Check sheet for the drawn part. Datum: minimum x, y, z corner. Units: mm. A direction names the side the tool comes from. Coordinates: 2 decimals unless noted, no trailing zeros. Order: outer loops, then holes, each group sorted by start corner. A loop starts at its lowest first (then second) coordinate and runs counter-clockwise, first axis right, second up. Notation, with made-up numbers: M 69.5,23 L 102.5,23 A30 cw 102.5,50 Z; hole C -23,-8.75 d8. An arc over 180 degrees is marked long. Answer in a Markdown table with one row per item. Add a question column.
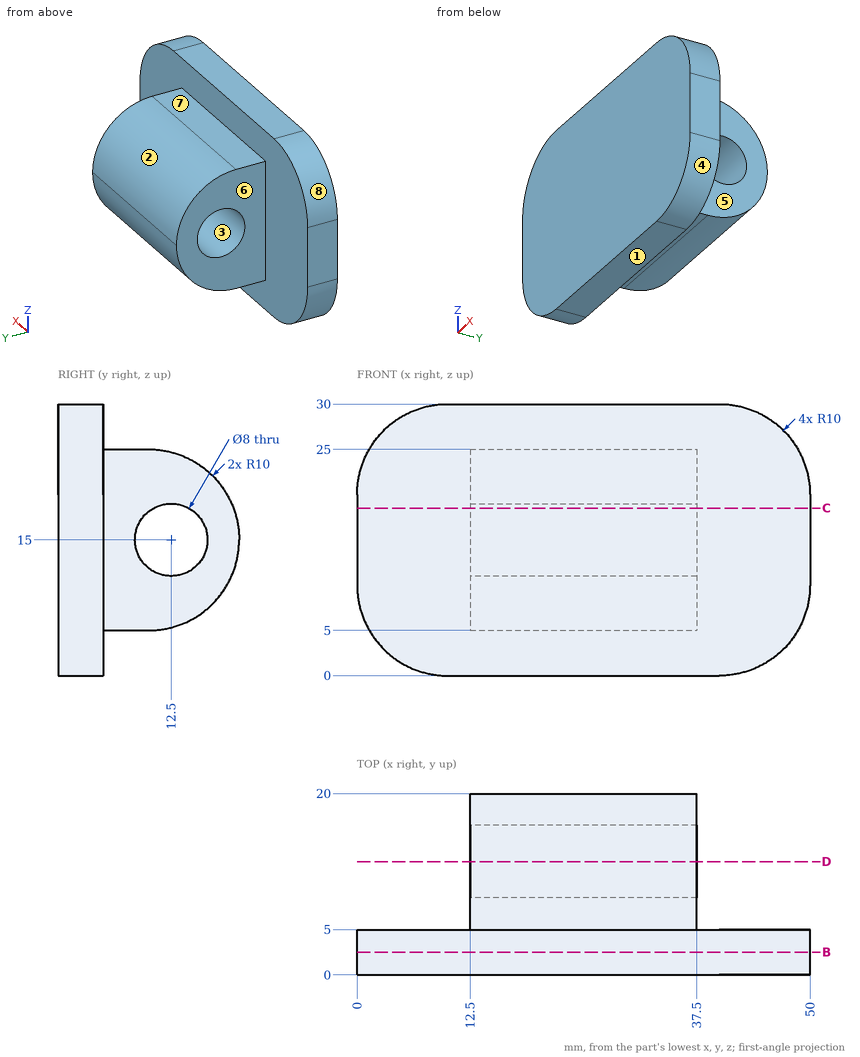
1. Scan lines: line 1 (Y direction, x = 18.25, z = 15); line 2 (X direction, y = 13, z = 9.5); line 3 (Y direction, x = 47, z = 17). Record each from-to range of solid material in increasing order.
2. Section check B-B on y = 2.5. Enter the section's corners in (x, z), then the cut area to 3 significant figures.
3. Section check D-D on y = 12.5. Enter the section's corners in (x, z), then the cut area to 3 significant figures.
4. Release check for a two-part mould opening along Y. For the marked faces 1, 2 and 3 record: released by +Y, released by -Y, zero draft, split by the parting line, or undercut.
5. Section check C-C on z = 18.5. Enter the section's corners in (x, y), then the cut area to 3 significant figures.
6. Go/stop test with flat-tipped pins: pin 1 Ø10 at (x, y) = (5.5, 10.5) entering from +Z; pin 2 Ø4 at (y, z) = (9, 20.5) entering from -X; pin 3 Ø1.5 at (x, y) = (31, 7.5) entering from +Z; pin 4 Ø7.5 at (y, z) = (9, 15.5) entering from +X. Record where each tip stops, or that it passes through.
7. Set-up check for the marked faces 4, 5, 6, 7 and 8: record each of +Z, -Z, +X, -X, +Y, -Y from which the full face is reachable in a straight line by a thin tool's end or side.
Result sheet:
| question | item | result |
|---|---|---|
| 1 | line 1 | 0 to 8.5, 16.5 to 20 |
| 1 | line 2 | 12.5 to 37.5 |
| 1 | line 3 | 0 to 5 |
| 2 | outline | M 0,10 A10 ccw 10,0 L 40,0 A10 ccw 50,10 L 50,20 A10 ccw 40,30 L 10,30 A10 ccw 0,20 Z |
| 2 | area | 1,410 mm^2 |
| 3 | outline | M 12.5,5.32 L 37.5,5.32 L 37.5,11 L 12.5,11 Z; M 12.5,19 L 37.5,19 L 37.5,24.68 L 12.5,24.68 Z |
| 3 | area | 284 mm^2 |
| 4 | face 1 | zero draft |
| 4 | face 2 | released by +Y |
| 4 | face 3 | undercut |
| 5 | outline | M 0,0 L 50,0 L 50,5 L 37.5,5 L 37.5,10.56 L 12.5,10.56 L 12.5,5 L 0,5 Z; M 12.5,14.44 L 37.5,14.44 L 37.5,19.37 L 12.5,19.37 Z |
| 5 | area | 512 mm^2 |
| 6 | pin 1 | through |
| 6 | pin 2 | x = 12.5 |
| 6 | pin 3 | z = 25 |
| 6 | pin 4 | x = 37.5 |
| 7 | face 4 | -Z, +X, +Y, -Y |
| 7 | face 5 | +Z, -Z, +X, +Y |
| 7 | face 6 | +Z, -Z, -X, +Y |
| 7 | face 7 | +Z, +X, -X, +Y |
| 7 | face 8 | +Z, -X, +Y, -Y |
